The figure shows three views and two pictorial views of one solid part (mm, origin at its lowest corner). Answer the questions. Give positions to 0.01 mm unless a question says otherwise; leave off trailing zeros. Order: outer loops, then holes, each group sorted by start corner. A loop starts at its lowest first (then second) coordinate and runs counter-clockwise, first axis right, second up. Notation, with made-up numbers: M -7,-38 L 4,-38 A36 ccw 4,-1 Z; hole C -7,-18 d8. An arc over 180 degrees is marked long. Write item = value, one per line. Start each with the question number.
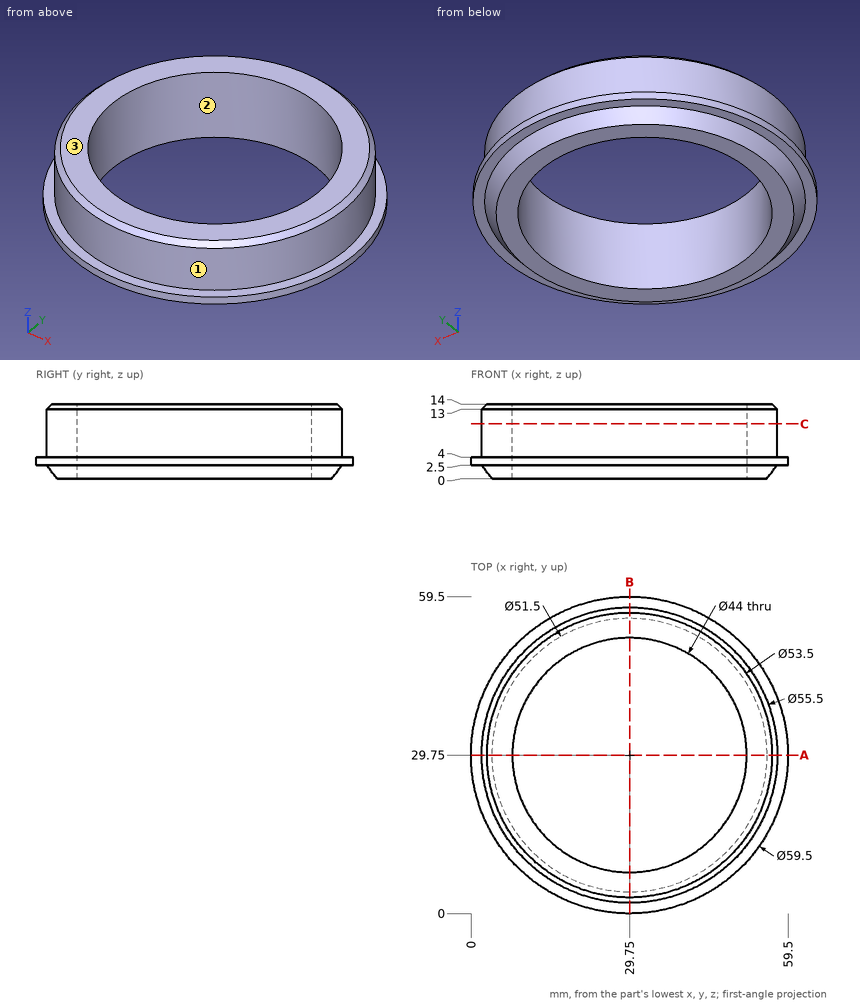
1) Find section A-A on y = 29.75. Determine the outline of the cut face in (x, z), plus the area to 3 significant figures.
2) Find the intervals of material crossed by probe 1 along Y at (x, z) = (29.75, 4.25); probe 2 along Y at (x, z) = (49.5, 10.5); probe 3 along X at (y, z) = (32, 12), in increasing order. Write a range as [from, to].
3) Find section C-C on z = 10.25. Determine the outline of the cut face in (x, y).
4) Each of these flat-tipped pins is pushed along its axis until it touches: P1, Ø1.5, axis at y = 33, z = 4.5, coming from the +X side; P2, Ø6, axis at x = 28, z = 10, coming from the -Y side; P3, Ø8, axis at y = 48.5, z = 10, coming from the -X side. Where does it stop, or does it pass through?
5) For a pull along X with two mould halves and no side action, classify the marked faces 1, 2 and 3 as pulls with the +X half, pulls with the -X half, needs draft (parallel to the pull), parting line crosses it, or undercut.
Numbers:
q1.outline = M 0,2.5 L 2,2.5 L 4,0 L 7.75,0 L 7.75,14 L 3,14 L 2,13 L 2,4 L 0,4 Z; M 51.75,0 L 55.5,0 L 57.5,2.5 L 59.5,2.5 L 59.5,4 L 57.5,4 L 57.5,13 L 56.5,14 L 51.75,14 Z
q1.area = 161 mm2
q2.probe_1 = [2, 7.75], [51.75, 57.5]
q2.probe_2 = [10.26, 20.06], [39.44, 49.24]
q2.probe_3 = [2.09, 7.87], [51.63, 57.41]
q3.outline = C 29.75,29.75 d55.5; hole C 29.75,29.75 d44
q4.P1 = 59.38
q4.P2 = 2
q4.P3 = 6.24
q5.face_1 = parting line crosses it
q5.face_2 = undercut
q5.face_3 = needs draft
